Geometry check sheet. Reference: the model listing, model coordinates, mm. Round coordinates to 2 decimals unless told otherwise and drop trailing zeros. Order: outer loops, then holes, each group sorted by start corner. A loop starts at its lowest first (then second) coordinate and runs counter-clockwise, first axis right, second up. Notation, with made-up numbers: M 80,-22.75 L 115,-22.75 A11 cw 115,-18.75 Z; hole C -19,0 d6. An arc over 180 degrees is marked long. Return JSON: item names as keys, results as strings. Group by question number.
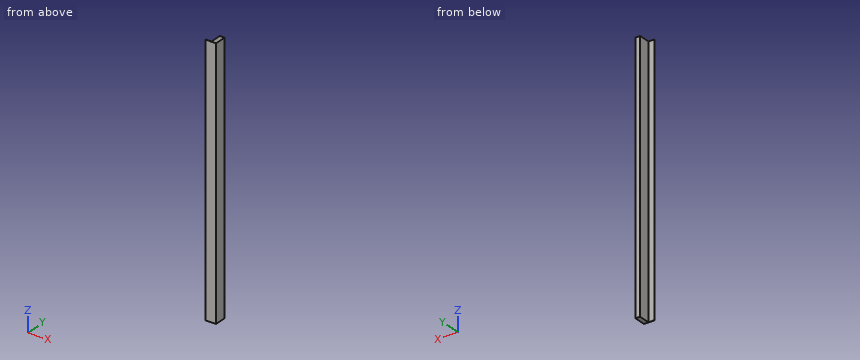
```python
from build123d import *

# Parameters (mm, degrees)
SKETCH1_W           = 12.7
SKETCH1_H           = 30.48
BOSS_EXTRUDE1_DEPTH = 558.8
SKETCH2_OUTSIDE_W   = 126.654
SKETCH2_OUTSIDE_H   = 144.434
SKETCH2_OUTSIDE_W_2 = 10.16
SKETCH2_OUTSIDE_H_2 = 25.4
CUT_EXTRUDE1_DEPTH  = 560.043844524
SKETCH3_W           = 12.7
SKETCH3_H           = 0.635
BOSS_EXTRUDE2_DEPTH = 558.8


with BuildPart() as part:
    # Sketch1 → Boss-Extrude1 (new body)
    with BuildSketch(Plane.XY):
        Rectangle(SKETCH1_W, SKETCH1_H)
    extrude(amount=BOSS_EXTRUDE1_DEPTH)

    # Sketch2 outside → Cut-Extrude1 (cut, through all)
    with BuildSketch(Plane.XY.offset(558.8)):
        Rectangle(SKETCH2_OUTSIDE_W, SKETCH2_OUTSIDE_H)
        with Locations((-1.27, 0)):
            Rectangle(SKETCH2_OUTSIDE_W_2, SKETCH2_OUTSIDE_H_2, mode=Mode.SUBTRACT)
    extrude(amount=-CUT_EXTRUDE1_DEPTH, mode=Mode.SUBTRACT)

    # Sketch3 → Boss-Extrude2 (add)
    with BuildSketch(Plane.XY):
        with Locations((-12.7, -12.3825)):
            Rectangle(SKETCH3_W, SKETCH3_H)
    extrude(amount=BOSS_EXTRUDE2_DEPTH)


solid = part.part
```
Q1. Material ranges on line 1 along X through (y, z) = (-4, 447.5); line 2 along Y through (x, z) = (-9.75, 171) (3 decimals), recorded low to high.
Q2. Section check C-C on y = 2. Record the cut outline in (x, z).
Q3. Section check A-A on z = 217. Record the cut outline in (x, y) (3 decimals).
Q4. Depth check by flat-ended pin: pin 1 Ø1.5 at (y, z) = (-2.5, 232) entering from -X. Enter the tip coordinate at first touch or a pass-through.
Q5. Section check B-B on x = -12. Record the cut outline in (y, z) (3 decimals), plus the area to 3 significant figures.
Geometry check:
{
 "1": {"line 1": "x = -6.35 to 3.81", "line 2": "y = -12.7 to -12.065"},
 "2": {"outline": "M -6.35,0 L 3.81,0 L 3.81,558.8 L -6.35,558.8 Z"},
 "3": {"outline": "M -19.05,-12.7 L 3.81,-12.7 L 3.81,12.7 L -6.35,12.7 L -6.35,-12.065 L -19.05,-12.065 Z"},
 "4": {"pin 1": "stops at x = -6.35"},
 "5": {"outline": "M -12.7,0 L -12.065,0 L -12.065,558.8 L -12.7,558.8 Z", "area": "355 mm^2"}
}
